Build history of the part. All positions in model axes, mm. Face numbers are marked on the shaded views. A direction names the side the tool comes from. Round coordinates to 2 decimals unless told otherwise and drop trailing zeros. Loops run counter-clockwise (first coordinate to the right, second up) from the corner with the lowest first, then second, coordinate; pieces in that order, holes last. Notation, with made-up numbers: (49, -15.5) - (96, -15.5) arc R14 ccw to (96, 3.5) - close; hole circle Ø8 at (-3.5, 21.5). An arc over 180 degrees is marked (long way). Put each result on its own line as item: value. Start each with the question number.
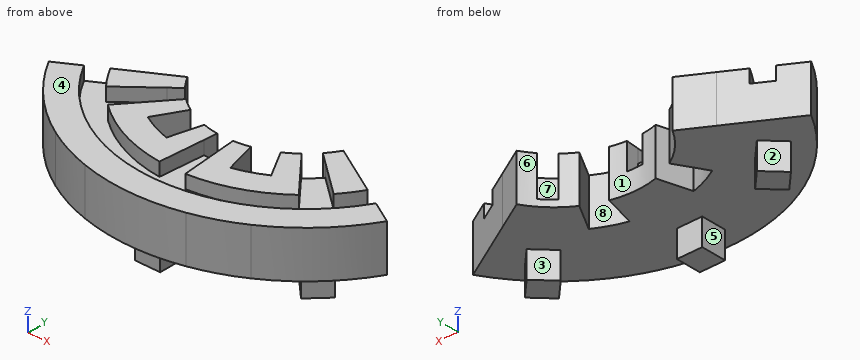
from build123d import *

# Parameters (mm, degrees)
F0_W     = 3.8
F0_H     = 3.8
F0_R     = 1
F1_DEPTH = 7
F2_DEPTH = 4
F5_DEPTH = 2
F6_DEPTH = 2
F7_DEPTH = 4
F8_DEPTH = 6


with BuildPart() as f1:
    # F0 (on Top) → F1 (new body)
    with BuildSketch(Plane.XY):
        with BuildLine():
            ThreePointArc((14.6437525, -25.3637233435), (20.7093933895, -20.7093933895), (25.3637233435, -14.6437525))
            Line((25.3637233435, -14.6437525), (16.0434713454, -9.2627025))
            ThreePointArc((16.0434713454, -9.2627025), (13.0994394997, -13.0994394997), (9.2627025, -16.0434713454))
            Line((9.2627025, -16.0434713454), (14.6437525, -25.3637233435))
        make_face()
        Polygon((17.2713695087, -14.5843637402), (19.9583752772, -17.2713695087), (17.2713695087, -19.9583752772), (14.5843637402, -17.2713695087), align=None, mode=Mode.SUBTRACT)
        Polygon((17.2713695087, -19.9583752772), (19.9583752772, -17.2713695087), (17.2713695087, -14.5843637402), (14.5843637402, -17.2713695087), align=None)
        with BuildLine():
            ThreePointArc((9.2627025, -16.0434713454), (13.0994394997, -13.0994394997), (16.0434713454, -9.2627025))
            Line((16.0434713454, -9.2627025), (11.6913429511, -6.75))
            ThreePointArc((11.6913429511, -6.75), (9.545941546, -9.545941546), (6.75, -11.6913429511))
            Line((6.75, -11.6913429511), (9.2627025, -16.0434713454))
        make_face()
        with BuildLine():
            ThreePointArc((7.5801640775, -28.2895574671), (11.2078429388, -27.0581264278), (14.6437525, -25.3637233435))
            Line((14.6437525, -25.3637233435), (9.2627025, -16.0434713454))
            ThreePointArc((9.2627025, -16.0434713454), (7.0893655714, -17.115242511), (4.7947276322, -17.894167132))
            Line((4.7947276322, -17.894167132), (7.5801640775, -28.2895574671))
        make_face()
        with BuildLine():
            Line((-4.7947276322, -17.894167132), (-7.5801640775, -28.2895574671))
            ThreePointArc((-7.5801640775, -28.2895574671), (0, -29.287505), (7.5801640775, -28.2895574671))
            Line((7.5801640775, -28.2895574671), (4.7947276322, -17.894167132))
            ThreePointArc((4.7947276322, -17.894167132), (0, -18.525405), (-4.7947276322, -17.894167132))
        make_face()
        with Locations((0, -24.425405)):
            Rectangle(F0_W, F0_H, mode=Mode.SUBTRACT)
        with Locations((0, -24.425405)):
            Rectangle(F0_W, F0_H)
        with Locations((0, -24.425405)):
            Circle(F0_R, mode=Mode.SUBTRACT)
        with Locations((0, -24.425405)):
            Circle(F0_R)
        with BuildLine():
            Line((-3.4940571089, -13.0399986549), (-4.7947276322, -17.894167132))
            ThreePointArc((-4.7947276322, -17.894167132), (0, -18.525405), (4.7947276322, -17.894167132))
            Line((4.7947276322, -17.894167132), (3.4940571089, -13.0399986549))
            ThreePointArc((3.4940571089, -13.0399986549), (0, -13.5), (-3.4940571089, -13.0399986549))
        make_face()
        with BuildLine():
            Line((-9.2627025, -16.0434713454), (-14.6437525, -25.3637233435))
            ThreePointArc((-14.6437525, -25.3637233435), (-11.2078429388, -27.0581264278), (-7.5801640775, -28.2895574671))
            Line((-7.5801640775, -28.2895574671), (-4.7947276322, -17.894167132))
            ThreePointArc((-4.7947276322, -17.894167132), (-7.0893655714, -17.115242511), (-9.2627025, -16.0434713454))
        make_face()
        with BuildLine():
            Line((-16.0434713454, -9.2627025), (-25.3637233435, -14.6437525))
            ThreePointArc((-25.3637233435, -14.6437525), (-20.7093933895, -20.7093933895), (-14.6437525, -25.3637233435))
            Line((-14.6437525, -25.3637233435), (-9.2627025, -16.0434713454))
            ThreePointArc((-9.2627025, -16.0434713454), (-13.0994394997, -13.0994394997), (-16.0434713454, -9.2627025))
        make_face()
        Polygon((-14.5843637402, -17.2713695087), (-17.2713695087, -19.9583752772), (-19.9583752772, -17.2713695087), (-17.2713695087, -14.5843637402), align=None, mode=Mode.SUBTRACT)
        Polygon((-19.9583752772, -17.2713695087), (-17.2713695087, -19.9583752772), (-14.5843637402, -17.2713695087), (-17.2713695087, -14.5843637402), align=None)
        with BuildLine():
            Line((-11.6913429511, -6.75), (-16.0434713454, -9.2627025))
            ThreePointArc((-16.0434713454, -9.2627025), (-13.0994394997, -13.0994394997), (-9.2627025, -16.0434713454))
            Line((-9.2627025, -16.0434713454), (-6.75, -11.6913429511))
            ThreePointArc((-6.75, -11.6913429511), (-9.545941546, -9.545941546), (-11.6913429511, -6.75))
        make_face()
    extrude(amount=F1_DEPTH)

    # F0 (on Top) → F2 (join)
    with BuildSketch(Plane.XY):
        Polygon((17.2713695087, -19.9583752772), (19.9583752772, -17.2713695087), (17.2713695087, -14.5843637402), (14.5843637402, -17.2713695087), align=None)
        with Locations((0, -24.425405)):
            Rectangle(F0_W, F0_H)
        with Locations((0, -24.425405)):
            Circle(F0_R, mode=Mode.SUBTRACT)
        with Locations((0, -24.425405)):
            Circle(F0_R)
        Polygon((-19.9583752772, -17.2713695087), (-17.2713695087, -19.9583752772), (-14.5843637402, -17.2713695087), (-17.2713695087, -14.5843637402), align=None)
    extrude(amount=-F2_DEPTH)

    # F4 (on offset) → F5 (cut)
    with BuildSketch(Plane.XY.offset(7)):
        with BuildLine():
            Line((-11.8736888683, -9.9632079501), (-17.0732193562, -14.3261320648))
            ThreePointArc((-17.0732193562, -14.3261320648), (-15.7596459212, -15.7596459212), (-14.3261320648, -17.0732193562))
            Line((-14.3261320648, -17.0732193562), (-9.9632079501, -11.8736888683))
            ThreePointArc((-9.9632079501, -11.8736888683), (-10.9601551084, -10.9601551084), (-11.8736888683, -9.9632079501))
        make_face()
        with BuildLine():
            Line((-1.3509140126, -15.4410178204), (-1.9424840523, -22.2026943147))
            ThreePointArc((-1.9424840523, -22.2026943147), (0, -22.287505), (1.9424840523, -22.2026943147))
            Line((1.9424840523, -22.2026943147), (1.3509140126, -15.4410178204))
            ThreePointArc((1.3509140126, -15.4410178204), (0, -15.5), (-1.3509140126, -15.4410178204))
        make_face()
        with BuildLine():
            ThreePointArc((14.3261320648, -17.0732193562), (15.7596459212, -15.7596459212), (17.0732193562, -14.3261320648))
            Line((17.0732193562, -14.3261320648), (11.8736888683, -9.9632079501))
            ThreePointArc((11.8736888683, -9.9632079501), (10.9601551084, -10.9601551084), (9.9632079501, -11.8736888683))
            Line((9.9632079501, -11.8736888683), (14.3261320648, -17.0732193562))
        make_face()
        with BuildLine():
            Line((-19.301545517, -11.1437525), (-21.8996217283, -12.6437525))
            ThreePointArc((-21.8996217283, -12.6437525), (0, -25.287505), (21.8996217283, -12.6437525))
            Line((21.8996217283, -12.6437525), (19.301545517, -11.1437525))
            ThreePointArc((19.301545517, -11.1437525), (18.2568552829, -12.7835876931), (17.0732193562, -14.3261320648))
            ThreePointArc((17.0732193562, -14.3261320648), (15.7596459212, -15.7596459212), (14.3261320648, -17.0732193562))
            ThreePointArc((14.3261320648, -17.0732193562), (8.5290589123, -20.5909697002), (1.9424840523, -22.2026943147))
            ThreePointArc((1.9424840523, -22.2026943147), (0, -22.287505), (-1.9424840523, -22.2026943147))
            ThreePointArc((-1.9424840523, -22.2026943147), (-8.5290589123, -20.5909697002), (-14.3261320648, -17.0732193562))
            ThreePointArc((-14.3261320648, -17.0732193562), (-15.7596459212, -15.7596459212), (-17.0732193562, -14.3261320648))
            ThreePointArc((-17.0732193562, -14.3261320648), (-18.2568552829, -12.7835876931), (-19.301545517, -11.1437525))
        make_face()
    extrude(amount=-F5_DEPTH, mode=Mode.SUBTRACT)

    # F4 (on offset) → F6 (cut)
    with BuildSketch(Plane.XY.offset(7)):
        with BuildLine():
            Line((-10.3415999821, -8.6776327308), (-11.8736888683, -9.9632079501))
            ThreePointArc((-11.8736888683, -9.9632079501), (-10.9601551084, -10.9601551084), (-9.9632079501, -11.8736888683))
            Line((-9.9632079501, -11.8736888683), (-8.6776327308, -10.3415999821))
            ThreePointArc((-8.6776327308, -10.3415999821), (-9.545941546, -9.545941546), (-10.3415999821, -8.6776327308))
        make_face()
    extrude(amount=-F6_DEPTH, mode=Mode.SUBTRACT)

    # F4 (on offset) → F7 (cut)
    with BuildSketch(Plane.XY.offset(7)):
        with BuildLine():
            Line((-1.1766025271, -13.4486284242), (-1.3509140126, -15.4410178204))
            ThreePointArc((-1.3509140126, -15.4410178204), (0, -15.5), (1.3509140126, -15.4410178204))
            Line((1.3509140126, -15.4410178204), (1.1766025271, -13.4486284242))
            ThreePointArc((1.1766025271, -13.4486284242), (0, -13.5), (-1.1766025271, -13.4486284242))
        make_face()
    extrude(amount=-F7_DEPTH, mode=Mode.SUBTRACT)

    # F4 (on offset) → F8 (cut)
    with BuildSketch(Plane.XY.offset(7)):
        with BuildLine():
            ThreePointArc((9.9632079501, -11.8736888683), (10.9601551084, -10.9601551084), (11.8736888683, -9.9632079501))
            Line((11.8736888683, -9.9632079501), (10.3415999821, -8.6776327308))
            ThreePointArc((10.3415999821, -8.6776327308), (9.545941546, -9.545941546), (8.6776327308, -10.3415999821))
            Line((8.6776327308, -10.3415999821), (9.9632079501, -11.8736888683))
        make_face()
    extrude(amount=-F8_DEPTH, mode=Mode.SUBTRACT)


solid = f1.part
1) Slice it at D-D, the plane y = -23. Write the cut outline in (x, z).
2) Slice it at C-C, the plane x = 3. Write the cut outline in (y, z), and give its area (3 significant figures).
3) Drop flat-ended pins along their axis: pin 1 Ø3 at (x, z) = (-16, 0.5) entering from -Y; pin 2 Ø2 at (y, z) = (-24, 1.5) entering from -X; pin 3 Ø2.5 at (x, y) = (11, -9.5) entering from +Z; pin 4 Ø3 at (y, z) = (-25, -2.5) entering from -X. Give the stop position or say it passes through.
4) Which spindle directions (+Z, -Z, +X, -X, +Y, -Y) get a long thin tool onto all of the face, cutting with end or side? Do the marked faces 5, 6, 7 and 8. Say none if no direction does.
5) Drill centre lines: line 1 (X direction, y = -18.5, z = 5.25); line 2 (Z direction, x = 14.5, y = -19.75); line 3 (X direction, y = -16.5, z = 0.5). Where is each one in solid material? Low to high. Write a range as [from, to].
6) Slice it at B-B, the plane z = 2.5. Write the cut outline in (x, y), and give its area (3 significant figures).
7) Slice it at A-A, the plane z = -2. Write the cut outline in (x, y).
8) Pull direction X, two halves, no side cores. Call the marked faces 1, 2, 3 and 4: pulls with the +X half, pulls with the -X half, needs draft (parallel to the pull), parting line crosses it, or undercut.
Taken from the geometry:
1. outline: (-18.13, 0) - (-1.9, 0) - (-1.9, -4) - (1.9, -4) - (1.9, 0) - (18.13, 0) - (18.13, 7) - (10.51, 7) - (10.51, 5) - (-10.51, 5) - (-10.51, 7) - (-18.13, 7) - close
2. outline: (-29.13, 0) - (-13.16, 0) - (-13.16, 7) - (-22.08, 7) - (-22.08, 5) - (-25.11, 5) - (-25.11, 7) - (-29.13, 7) - close
2. area: 106 mm2
3. pin 1: stops at y = -25.45
3. pin 2: stops at x = -18.13
3. pin 3: stops at z = 7
3. pin 4: stops at x = -1.9
4. face 5: -Z, -X, +Y, -Y
4. face 6: +Z, -Z, +Y
4. face 7: +Z
4. face 8: +Z, -Z
5. line 1: x = [-22.7, -17.24], [-12.43, -1.62], [1.62, 12.43], [17.24, 22.7]
5. line 2: z = [0, 5]
5. line 3: x = [-24.2, -8.42], [-4.42, 4.42], [8.42, 24.2]
6. outline: (-25.36, -14.64) arc R29.29 ccw to (25.36, -14.64) - (11.69, -6.75) arc R13.5 cw to (10.34, -8.68) - (11.87, -9.96) arc R15.5 cw to (9.96, -11.87) - (8.68, -10.34) arc R13.5 cw to (6.75, -11.69) - (9.26, -16.04) arc R18.53 cw to (4.79, -17.89) - (3.49, -13.04) arc R13.5 cw to (-3.49, -13.04) - (-4.79, -17.89) arc R18.53 cw to (-9.26, -16.04) - (-6.75, -11.69) arc R13.5 cw to (-11.69, -6.75) - close
6. area: 660 mm2
7. outline: (-19.96, -17.27) - (-17.27, -19.96) - (-14.58, -17.27) - (-17.27, -14.58) - close; (-1.9, -26.33) - (1.9, -26.33) - (1.9, -22.53) - (-1.9, -22.53) - close; (14.58, -17.27) - (17.27, -19.96) - (19.96, -17.27) - (17.27, -14.58) - close
8. face 1: undercut
8. face 2: pulls with the -X half
8. face 3: undercut
8. face 4: needs draft
